Source: CAD feature listing. Evaluate the final solid. Frame: model axes, mm. A direction names the side the tool comes from. Coordinates: 2 decimals unless noted, no trailing zeros. Order: outer loops, then holes, each group sorted by start corner. A loop starts at its lowest first (then second) coordinate and runs counter-clockwise, first axis right, second up. Notation, with made-up numbers: (35, -7) -> (39, -7) arc R25 cw to (39, 27) -> close; hole circle Ø8 at (84, 43.5). An arc over 180 degrees is marked (long way). Put each result on its own line as item: value.
from build123d import *

# Parameters (mm, degrees)
SKETCH_1_R              = 11.25
SKETCH_1_R_2            = 4.25
EXTRUDE_1_DEPTH         = 13
SKETCH_2_W              = 20
SKETCH_2_H              = 20
CUT_EXTRUDE_1_DEPTH     = 108.071751643
CUT_EXTRUDE1_DEPTH      = 71.08823011
CUT_EXTRUDE1_DEPTH_BACK = 71.08823011
SKETCH1_R               = 2.75


with BuildPart() as part:
    # Эскиз1 → Бобышка-Вытянуть1 (new, symmetric)
    with BuildSketch(Plane(origin=(0, 0, 0), x_dir=(1, 0, 0), z_dir=(0, 1, 0))):
        Polygon((-48, -10.5), (48, -10.5), (48, 10.5), (35.224644777, 45.6), (0, 45.6), (-35.224644777, 45.6), (-48, 10.5), align=None)
        with Locations(Location((0, 30.6, 0), (0, 0, 90))):
            Circle(SKETCH_1_R, mode=Mode.SUBTRACT)
        with Locations(Location((-30, 30.6, 0), (0, 0, 90))):
            Circle(SKETCH_1_R_2, mode=Mode.SUBTRACT)
        with Locations(Location((30, 30.6, 0), (0, 0, 90))):
            Circle(SKETCH_1_R_2, mode=Mode.SUBTRACT)
    extrude(amount=EXTRUDE_1_DEPTH, both=True)

    # Эскиз2 → Вырез-Вытянуть1 (cut, through all)
    with BuildSketch(Plane.ZY.offset(48)):
        with Locations((0.5, 0)):
            Rectangle(SKETCH_2_W, SKETCH_2_H)
    extrude(amount=-CUT_EXTRUDE_1_DEPTH, mode=Mode.SUBTRACT)

    # Sketch1 → Cut-Extrude1 (cut, two sides: drawn at the far end of the back side and taken through both)
    with BuildSketch(Plane.XZ.offset(-10).offset(-CUT_EXTRUDE1_DEPTH_BACK)):
        with Locations(Location((-33, 0.5, 0), (0, 0, 270))):
            Circle(SKETCH1_R)
        with Locations(Location((33, 0.5, 0), (0, 0, 270))):
            Circle(SKETCH1_R)
    extrude(amount=CUT_EXTRUDE1_DEPTH + CUT_EXTRUDE1_DEPTH_BACK, mode=Mode.SUBTRACT)


solid = part.part
1. Cut plane A-A on z = 0.5. Output: boundary loops of the cut face in (x, y), plus the area to 3 significant figures.
Numbers:
outline: (-48, -13) -> (-35.75, -13) -> (-35.75, -10) -> (-48, -10) -> close; (-48, 10) -> (-35.75, 10) -> (-35.75, 13) -> (-48, 13) -> close; (-30.25, -13) -> (30.25, -13) -> (30.25, -10) -> (-30.25, -10) -> close; (-30.25, 10) -> (30.25, 10) -> (30.25, 13) -> (-30.25, 13) -> close; (35.75, -13) -> (48, -13) -> (48, -10) -> (35.75, -10) -> close; (35.75, 10) -> (48, 10) -> (48, 13) -> (35.75, 13) -> close
area: 510 mm2
2. Ray query, line 1 along X through (y, z) = (12.45, 0.5); line 2 along Y through (x, z) = (-7.5, -8.5); line 3 along X through (y, z) = (3.75, -30.6). Return the intervals inside material, ascending.
Numbers:
line 1: x = -48 to -35.75, -30.25 to 30.25, 35.75 to 48
line 2: y = -13 to -10, 10 to 13
line 3: x = -40.68 to -34.25, -25.75 to -11.25, 11.25 to 25.75, 34.25 to 40.68
3. Cut plane B-B on x = 0. Output: boundary loops of the cut face in (y, z).
Numbers:
outline: (-13, -45.6) -> (13, -45.6) -> (13, -41.85) -> (-13, -41.85) -> close; (-13, -19.35) -> (13, -19.35) -> (13, 10.5) -> (10, 10.5) -> (10, -9.5) -> (-10, -9.5) -> (-10, 10.5) -> (-13, 10.5) -> close
4. Pull-direction query (X, two-part tool) for faces 1 (the cylindrical face through (-30.273, -11.479, 0.858)), 2 (the flat face through (-1, 10, 0)), 3 (the flat face through (-48, -1, -10)); classes: pulls with the +X half, pulls with the -X half, needs draft (parallel to the pull), parting line crosses it, or undercut.
Numbers:
face 1: undercut
face 2: needs draft
face 3: pulls with the -X half
5. Cut plane C-C on y = -1.5. Output: boundary loops of the cut face in (x, z), plus the area to 3 significant figures.
Numbers:
outline: (-48, -10.5) -> (-35.22, -45.6) -> (35.22, -45.6) -> (48, -10.5) -> (48, -9.5) -> (-48, -9.5) -> close; hole circle Ø8.5 at (-30, -30.6); hole circle Ø22.5 at (0, -30.6); hole circle Ø8.5 at (30, -30.6)
area: 2,510 mm2
6. Cut plane D-D on z = -30.6. Output: boundary loops of the cut face in (x, y).
Numbers:
outline: (-40.68, -13) -> (-34.25, -13) -> (-34.25, 13) -> (-40.68, 13) -> close; (-25.75, -13) -> (-11.25, -13) -> (-11.25, 13) -> (-25.75, 13) -> close; (11.25, -13) -> (25.75, -13) -> (25.75, 13) -> (11.25, 13) -> close; (34.25, -13) -> (40.68, -13) -> (40.68, 13) -> (34.25, 13) -> close
7. First-contact query: pin 1 (1.5 mm diameter, centred on x = -19, y = -3.5, fed in from +Z); pin 2 (4 mm diameter, centred on y = -4.5, z = -15.5, fed in from -X). Flat tips, straight axial feed; report the tip coordinate or a pass-through.
Numbers:
pin 1: stops at z = -9.5
pin 2: stops at x = -46.91
8. Set-up query: faces 4 (the flat face through (-1, -10, 0)), 5 (the cylindrical face through (-30.273, 11.521, 0.858)). Return all of +Z, -Z, +X, -X, +Y, -Y with unobstructed straight access to the full face (end or side cutting, diameter ignored); none if empty.
Numbers:
face 4: +Z, +X, -X
face 5: +Y, -Y
